The figure shows three views and two pictorial views of one solid part (mm, origin at its lowest corner). Answer the questions. Coordinates: 2 decimals unless noted, no trailing zeros. Loops run counter-clockwise (first coordinate to the right, second up) from the corner with the lowest first, then second, coordinate; pieces in that order, holes last. Notation, with made-up numbers: (7.25, -34.75) - (59.25, -34.75) arc R21 ccw to (59.25, -27.75) - close; hole circle Ø7 at (2.25, 53). An arc over 180 degrees is marked (long way). One line per question, with ' | ' between items.
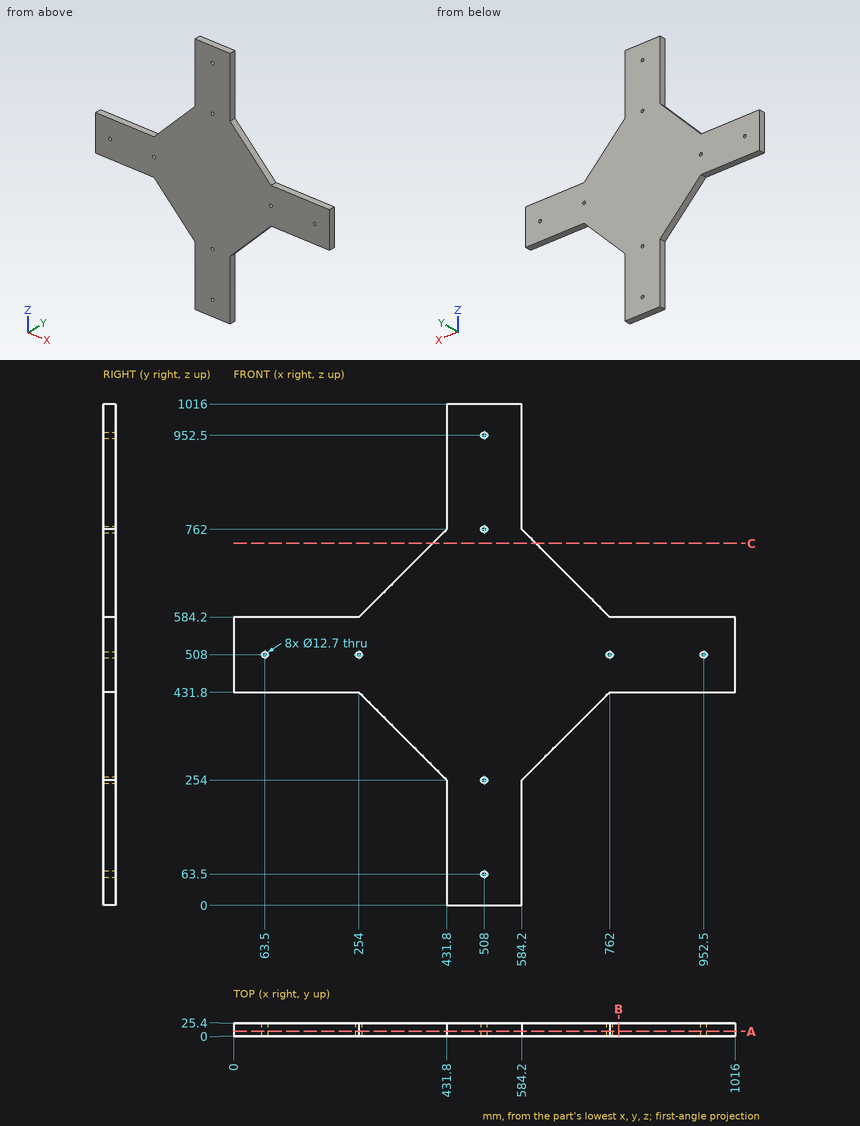
Item 1: Find section C-C, the plane z = 733.5. Write down the section's boundary in (x, y), plus the area to 3 significant figures.
Taken from the geometry:
outline: (403.3, 0) - (612.7, 0) - (612.7, 25.4) - (403.3, 25.4) - close | area: 5,320 mm2
Item 2: Find section B-B, the plane x = 780. Write down the section's boundary in (y, z), plus the area to 3 significant figures.
Taken from the geometry:
outline: (0, 431.8) - (25.4, 431.8) - (25.4, 584.2) - (0, 584.2) - close | area: 3,870 mm2
Item 3: Each of these flat-tipped pins is pushed along its axis until it touches: pin 1 Ø11.5 at (x, z) = (63.5, 508) entering from +Y; pin 2 Ø16.5 at (x, z) = (508, 254) entering from +Y; pin 3 Ø2 at (x, y) = (690, 14.5) entering from -Z; pin 4 Ø7.5 at (x, y) = (180.5, 17) entering from +Z. Where does it stop, or does it pass through?
Taken from the geometry:
pin 1: passes through | pin 2: stops at y = 25.4 | pin 3: stops at z = 358.8 | pin 4: stops at z = 584.2
Item 4: Find the intervals of material crossed by line 1 (X direction, y = 18.25, z = 508); line 2 (X direction, y = 8.25, z = 952.5), in increasing order. Write a range as [from, to].
Taken from the geometry:
line 1: x = [0, 57.15], [69.85, 247.65], [260.35, 755.65], [768.35, 946.15], [958.85, 1016] | line 2: x = [431.8, 501.65], [514.35, 584.2]
Item 5: Find section A-A, the plane y = 9.5. State how many separate pieces and enclosed holes the cut face has, plus the area to 3 significant figures.
Taken from the geometry:
separate pieces: 1 | enclosed holes: 8 | area: 349,000 mm2
